Here's how the part is built. I have some questions about the finished solid (model axes, mm). Face numbers are marked on the shaded views. A direction names the side the tool comes from. Round coordinates to 2 decimals unless told otherwise and drop trailing zeros. Order: outer loops, then holes, each group sorted by start corner. A loop starts at its lowest first (then second) coordinate and runs counter-clockwise, first axis right, second up. Notation, with made-up numbers: (35, 84.5) -> (41, 84.5) arc R17 cw to (41, 112.5) -> close; hole circle Ø8 at (77.5, 14). An arc over 180 degrees is marked (long way). Answer in a Markdown table with one row per item.
```python
from build123d import *

# Parameters (mm, degrees)
BOSS_EXTRUDE4_DEPTH = 30
SKETCH12_R          = 1.65
CUT_EXTRUDE1_DEPTH  = 162.652709488
BOSS_EXTRUDE5_DEPTH = 30
CIRPATTERN1_DEPTH   = 30
CUT_EXTRUDE2_START  = -30
CUT_EXTRUDE2_DEPTH  = 30


# Read off the part's stored shape, not the designer's step: CirPattern1
with BuildPart() as part:
    # Sketch5 → Boss-Extrude4 (new body)
    with BuildSketch(Plane.XY):
        with BuildLine():
            Line((0, 0), (0, 150.337121164))
            ThreePointArc((0, 150.337121164), (-1.473777529, 152.266652173), (-3.723089911, 151.352483739))
            ThreePointArc((-3.723089911, 151.352483739), (-34.4957159, 78.440037035), (-45, 0))
            Line((-45, 0), (0, 0))
        make_face()
        with BuildLine():
            Line((-1.6, 10), (-40.829955095, 10))
            ThreePointArc((-40.829955095, 10), (-30.304470107, 78.595490327), (-4, 142.815440342))
            ThreePointArc((-4, 142.815440342), (-2.559389376, 143.433276944), (-1.6, 142.193658833))
            Line((-1.6, 142.193658833), (-1.6, 10))
        make_face(mode=Mode.SUBTRACT)
    extrude(amount=BOSS_EXTRUDE4_DEPTH)

    # Sketch12 → Cut-Extrude1 (cut, through all)
    with BuildSketch(Plane.XY.offset(30)):
        with Locations((-40, 5)):
            Circle(SKETCH12_R)
        with Locations((-22.5, 5)):
            Circle(SKETCH12_R)
        with Locations((-5, 5)):
            Circle(SKETCH12_R)
    extrude(amount=-CUT_EXTRUDE1_DEPTH, mode=Mode.SUBTRACT)

    # Sketch13 → Boss-Extrude5 (add)
    with BuildSketch(Plane.XY.offset(30)):
        Polygon((-101.6, 127.193658833), (-1.6, 10), (-2.741055234, 9.026350704), (-102.741055234, 126.220009537), align=None)
    extrude(amount=-BOSS_EXTRUDE5_DEPTH)

    # CirPattern1 outline → CirPattern1 (add)
    with BuildSketch(Plane.XY):
        with BuildLine():
            Line((-101.6, 127.193658833), (-90.428627174, 114.101518276))
            Line((-90.428627174, 114.101518276), (-38.303740092, 62.831561128))
            ThreePointArc((-38.303740092, 62.831561128), (-38.115676892, 63.697596098), (-37.925040114, 64.563068197))
            Line((-37.925040114, 64.563068197), (-89.330082385, 115.124987119))
            Line((-89.330082385, 115.124987119), (-36.32594483, 71.390938936))
            ThreePointArc((-36.32594483, 71.390938936), (-36.125817446, 72.197508487), (-35.923442521, 73.003517048))
            Line((-35.923442521, 73.003517048), (-88.324919079, 116.240305842))
            Line((-88.324919079, 116.240305842), (-34.318662851, 79.086385123))
            ThreePointArc((-34.318662851, 79.086385123), (-34.107234191, 79.850856393), (-33.893772384, 80.614762447))
            Line((-33.893772384, 80.614762447), (-87.420787154, 117.438986195))
            Line((-87.420787154, 117.438986195), (-32.265940677, 86.200502345))
            ThreePointArc((-32.265940677, 86.200502345), (-32.04280883, 86.93581789), (-31.817782431, 87.670555864))
            Line((-31.817782431, 87.670555864), (-86.624567601, 118.711905496))
            Line((-86.624567601, 118.711905496), (-30.142720205, 92.940380431))
            ThreePointArc((-30.142720205, 92.940380431), (-29.906617894, 93.656921246), (-29.668703058, 94.372862284))
            Line((-29.668703058, 94.372862284), (-85.942320131, 120.049376062))
            Line((-85.942320131, 120.049376062), (-27.915909182, 99.471216899))
            ThreePointArc((-27.915909182, 99.471216899), (-27.664777337, 100.177924555), (-27.411868402, 100.883998196))
            Line((-27.411868402, 100.883998196), (-85.379237059, 121.441218934))
            Line((-85.379237059, 121.441218934), (-25.542932289, 105.93724151))
            ThreePointArc((-25.542932289, 105.93724151), (-25.273841569, 106.642396064), (-25.002966495, 107.346867111))
            Line((-25.002966495, 107.346867111), (-84.939603787, 122.876841346))
            Line((-84.939603787, 122.876841346), (-22.968102286, 112.477173218))
            ThreePointArc((-22.968102286, 112.477173218), (-22.677026174, 113.189036497), (-22.384114637, 113.900146519))
            Line((-22.384114637, 113.900146519), (-84.62676619, 124.345317346))
            Line((-84.62676619, 124.345317346), (-20.11610645, 119.238472696))
            ThreePointArc((-20.11610645, 119.238472696), (-19.797493538, 119.965945777), (-19.476943816, 120.692567512))
            Line((-19.476943816, 120.692567512), (-84.443105151, 125.835470945))
            Line((-84.443105151, 125.835470945), (-16.880634523, 126.394117549))
            ThreePointArc((-16.880634523, 126.394117549), (-16.526645472, 127.147574571), (-16.170553887, 127.900040194))
            Line((-16.170553887, 127.900040194), (-84.390018442, 127.335961174))
            Line((-84.390018442, 127.335961174), (-13.103676665, 134.167087417))
            ThreePointArc((-13.103676665, 134.167087417), (-12.702778891, 134.959651729), (-12.299521655, 135.751018152))
            Line((-12.299521655, 135.751018152), (-101.6, 127.193658833))
        make_face()
        with BuildLine():
            Line((-102.741055234, 126.220009537), (-101.6, 127.193658833))
            Line((-101.6, 127.193658833), (-102.806194023, 126.301977287))
            Line((-102.806194023, 126.301977287), (-41.773547865, 43.741994606))
            ThreePointArc((-41.773547865, 43.741994606), (-41.616374453, 44.788813456), (-41.455485097, 45.835067632))
            Line((-41.455485097, 45.835067632), (-88.817221598, 109.902159449))
            Line((-88.817221598, 109.902159449), (-102.741055234, 126.220009537))
        make_face()
        with BuildLine():
            ThreePointArc((-34.552670054, 61.246010298), (-34.736897582, 60.374196024), (-34.918483062, 59.501827625))
            Line((-34.918483062, 59.501827625), (-1.6, 26.729819964))
            Line((-1.6, 26.729819964), (-1.6, 28.833815738))
            Line((-1.6, 28.833815738), (-34.552670054, 61.246010298))
        make_face()
        with BuildLine():
            ThreePointArc((-32.504088687, 70.182186635), (-32.701856665, 69.372354972), (-32.897328567, 68.561966034))
            Line((-32.897328567, 68.561966034), (-1.6, 42.738342848))
            Line((-1.6, 42.738342848), (-1.6, 44.683028154))
            Line((-1.6, 44.683028154), (-32.504088687, 70.182186635))
        make_face()
        with BuildLine():
            ThreePointArc((-30.409038425, 78.217419283), (-30.619276495, 77.451282634), (-30.827444392, 76.684580908))
            Line((-30.827444392, 76.684580908), (-1.6, 56.57738912))
            Line((-1.6, 56.57738912), (-1.6, 58.398072333))
            Line((-1.6, 58.398072333), (-30.409038425, 78.217419283))
        make_face()
        with BuildLine():
            ThreePointArc((-28.252621221, 85.651327492), (-28.475582862, 84.915412953), (-28.696619797, 84.178918027))
            Line((-28.696619797, 84.178918027), (-1.6, 68.831992526))
            Line((-1.6, 68.831992526), (-1.6, 70.555872953))
            Line((-1.6, 70.555872953), (-28.252621221, 85.651327492))
        make_face()
        with BuildLine():
            ThreePointArc((-26.008808525, 92.702926401), (-26.245713404, 91.98652139), (-26.480779611, 91.269510972))
            Line((-26.480779611, 91.269510972), (-1.6, 79.916914254))
            Line((-1.6, 79.916914254), (-1.6, 81.565680547))
            Line((-1.6, 81.565680547), (-26.008808525, 92.702926401))
        make_face()
        with BuildLine():
            ThreePointArc((-23.641877477, 99.547029874), (-23.894816729, 98.840967037), (-24.145954739, 98.134261515))
            Line((-24.145954739, 98.134261515), (-1.6, 90.138691265))
            Line((-1.6, 90.138691265), (-1.6, 91.730222742))
            Line((-1.6, 91.730222742), (-23.641877477, 99.547029874))
        make_face()
        with BuildLine():
            ThreePointArc((-21.104819389, 106.336831732), (-21.376834174, 105.63265906), (-21.647040774, 104.92779057))
            Line((-21.647040774, 104.92779057), (-1.6, 99.733471356))
            Line((-1.6, 99.733471356), (-1.6, 101.283005621))
            Line((-1.6, 101.283005621), (-21.104819389, 106.336831732))
        make_face()
        with BuildLine():
            ThreePointArc((-18.335117992, 113.220669335), (-18.63044525, 112.509971124), (-18.923911862, 111.798502583))
            Line((-18.923911862, 111.798502583), (-1.6, 108.891312509))
            Line((-1.6, 108.891312509), (-1.6, 110.412286949))
            Line((-1.6, 110.412286949), (-18.335117992, 113.220669335))
        make_face()
        with BuildLine():
            ThreePointArc((-15.247010957, 120.35771417), (-15.571555811, 119.631419453), (-15.8941351, 118.90424961))
            Line((-15.8941351, 118.90424961), (-1.6, 117.772685809))
            Line((-1.6, 117.772685809), (-1.6, 119.27737853))
            Line((-1.6, 119.27737853), (-15.247010957, 120.35771417))
        make_face()
        with BuildLine():
            ThreePointArc((-11.717737877, 127.936858719), (-12.079928782, 127.184359789), (-12.439981613, 126.430835503))
            Line((-12.439981613, 126.430835503), (-1.6, 126.520466904))
            Line((-1.6, 126.520466904), (-1.6, 128.020518181))
            Line((-1.6, 128.020518181), (-11.717737877, 127.936858719))
        make_face()
        with BuildLine():
            ThreePointArc((-7.562004039, 136.204998257), (-7.974393837, 135.412784341), (-8.384376146, 134.61932184))
            Line((-8.384376146, 134.61932184), (-1.6, 135.269445395))
            Line((-1.6, 135.269445395), (-1.6, 136.776316706))
            Line((-1.6, 136.776316706), (-7.562004039, 136.204998257))
        make_face()
        Polygon((0, 27.260058248), (0, 25.156062475), (7.181716143, 18.092137745), (8.23357019, 19.161531528), align=None)
        Polygon((0, 136.929639232), (0, 135.422767921), (51.900153262, 140.396182044), (51.757068846, 141.889342065), align=None)
        Polygon((0, 128.03374793), (0, 126.533696654), (52.466714553, 126.967522588), (52.454312086, 128.467471313), align=None)
        Polygon((0, 119.150718045), (0, 117.646025324), (51.860735117, 113.540584165), (51.979108991, 115.035906079), align=None)
        Polygon((0, 110.143784999), (0, 108.622810558), (50.086826826, 100.217553884), (50.335076143, 101.696868684), align=None)
        Polygon((0, 100.868435169), (0, 99.318900904), (47.158490191, 87.099828051), (47.534725625, 88.551877257), align=None)
        Polygon((0, 91.162807764), (0, 89.571276287), (43.098011623, 74.287240479), (43.599369795, 75.700973121), align=None)
        Polygon((0, 80.835632895), (0, 79.186866601), (37.936293815, 61.877302697), (38.558959087, 63.241959415), align=None)
        Polygon((0, 69.649668379), (0, 67.925787952), (31.712620558, 49.964461824), (32.451854069, 51.269656757), align=None)
        Polygon((0, 57.297342949), (0, 55.476659736), (24.474357761, 38.639381772), (25.3245335, 39.875181599), align=None)
        Polygon((0, 43.362858063), (0, 41.418172757), (16.276592976, 27.988253239), (17.231240592, 29.145252777), align=None)
        with BuildLine():
            Line((-16.829705211, 10), (-14.964333673, 10))
            Line((-14.964333673, 10), (-38.088693922, 41.280747301))
            ThreePointArc((-38.088693922, 41.280747301), (-38.23738412, 40.217865998), (-38.382194992, 39.154449216))
            Line((-38.382194992, 39.154449216), (-16.829705211, 10))
        make_face()
    extrude(amount=CIRPATTERN1_DEPTH)

    # Sketch14 → Cut-Extrude2 (cut)
    with BuildSketch(Plane.XY.offset(30).offset(CUT_EXTRUDE2_START)):
        Polygon((-129.094046134, -17.289617226), (770.905953866, -20.358672888), (773.974831033, 879.588983489), (-141.374926706, 882.710382774), align=None)
        with BuildLine():
            Line((-45, 0), (0, 0))
            Line((0, 0), (0, 150.337121164))
            ThreePointArc((0, 150.337121164), (-1.473777529, 152.266652173), (-3.723089911, 151.352483739))
            ThreePointArc((-3.723089911, 151.352483739), (-34.4957159, 78.440037035), (-45, 0))
        make_face(mode=Mode.SUBTRACT)
    extrude(amount=CUT_EXTRUDE2_DEPTH, mode=Mode.SUBTRACT)


solid = part.part
```
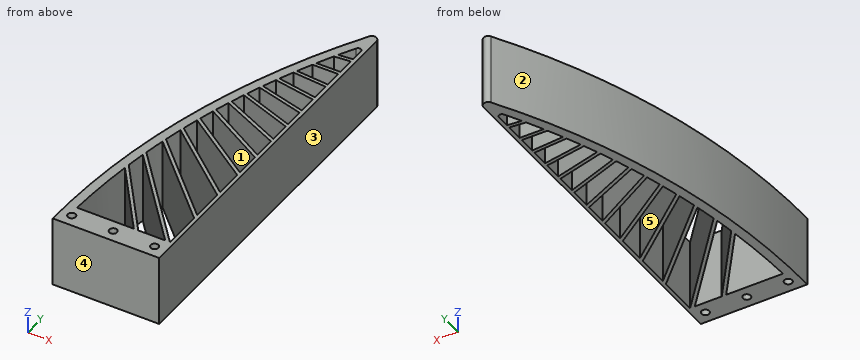
1. Suppose I cut it at C-C on z = 3.75. State how many separate pieces and enclosed holes the cut face has, then the cut area to 3 significant figures.
Numbers:
| item | result |
|---|---|
| separate pieces | 1 |
| enclosed holes | 17 |
| area | 1,790 mm2 |
2. Suppose I cut it at A-A on y = 5. Write out the boundary of the cut face in (x, z).
Numbers:
| item | result |
|---|---|
| outline | (-44.96, 0) -> (-41.65, 0) -> (-41.65, 30) -> (-44.96, 30) -> close; (-38.35, 0) -> (-24.15, 0) -> (-24.15, 30) -> (-38.35, 30) -> close; (-20.85, 0) -> (-6.65, 0) -> (-6.65, 30) -> (-20.85, 30) -> close; (-3.35, 0) -> (0, 0) -> (0, 30) -> (-3.35, 30) -> close |
3. For the marked faces 4 and 5, which set-ups out of +Z, -Z, +X, -X, +Y, -Y let a thin tool reach every point of the face, with its end or its side?
Numbers:
| item | result |
|---|---|
| face 4 | +Z, -Z, +X, -X, -Y |
| face 5 | +Z, -Z |
4. Suppose I cut it at D-D on y = 130. Write out the boundary of the cut face in (x, z), then the cut area to 3 significant figures.
Numbers:
| item | result |
|---|---|
| outline | (-15.16, 0) -> (-10.71, 0) -> (-10.71, 30) -> (-15.16, 30) -> close; (-1.6, 0) -> (0, 0) -> (0, 30) -> (-1.6, 30) -> close |
| area | 182 mm2 |
5. We'd pull the mould along Y, two halves only. Please class the marked faces 1, 2 and 3: released by +Y, released by -Y, zero draft, split by the parting line, or undercut.
Numbers:
| item | result |
|---|---|
| face 1 | undercut |
| face 2 | released by +Y |
| face 3 | zero draft |
6. For pin 1 Ø3.5 at (y, z) = (114.5, 10) entering from -X; pin 2 Ø4 at (y, z) = (36, 9) entering from -X; pin 3 Ø12 at (x, z) = (-24.5, 8.5) entering from +Y; pin 4 Ø2.5 at (x, y) = (-40, 5) entering from +Z, each with a flat end and sliding along its axis, tell me the tip position at first contact or that it passes through.
Numbers:
| item | result |
|---|---|
| pin 1 | stops at x = -22.86 |
| pin 2 | stops at x = -43.05 |
| pin 3 | stops at y = 122.88 |
| pin 4 | passes through |
7. Please list where these lines run through material, in increasing order: line 1 along X through (y, z) = (85, 28.75); line 2 along X through (y, z) = (62, 22.5); line 3 along X through (y, z) = (65, 14.25).
Numbers:
| item | result |
|---|---|
| line 1 | x = -32.63 to -27.1, -12.74 to -9.13, -1.6 to 0 |
| line 2 | x = -38.48 to -34.39, -24.94 to -22.59, -9.48 to -6.84, -1.6 to 0 |
| line 3 | x = -37.83 to -33.73, -28.58 to -26.22, -13.84 to -11.2, -1.6 to 0 |
8. Suppose I cut it at B-B on y = 32. Write out the boundary of the cut face in (x, z).
Numbers:
| item | result |
|---|---|
| outline | (-43.28, 0) -> (-39.25, 0) -> (-39.25, 30) -> (-43.28, 30) -> close; (-33.09, 0) -> (-31.23, 0) -> (-31.23, 30) -> (-33.09, 30) -> close; (-22.34, 0) -> (-20.37, 0) -> (-20.37, 30) -> (-22.34, 30) -> close; (-6.96, 0) -> (-4.82, 0) -> (-4.82, 30) -> (-6.96, 30) -> close; (-1.6, 0) -> (0, 0) -> (0, 30) -> (-1.6, 30) -> close |
